Autodesk Inventor part; units mm, degrees
ref_plane "YZ Plane" through (0, 0, 0) normal (1, 0, 0) x (0, 1, 0)
ref_plane "XZ Plane" through (0, 0, 0) normal (0, 1, 0) x (-1, 0, 0)
ref_plane "XY Plane" through (0, 0, 0) normal (0, 0, 1) x (1, 0, 0)
sketch "Sketch1" plane through (0, 0, 0) normal (0, 0, 1) x (1, 0, 0)
  line L0 (0, 0) -> (50.8, 0)
  line L1 (50.8, 0) -> (50.8, 107.95)
  line L2 (50.8, 107.95) -> (0, 107.95)
  line L3 (0, 107.95) -> (0, 0)
  dimension "d0" = 50.8
  dimension "d1" = 107.95
extrude "Plate1" add sketch "Sketch1" along normal blind 3.048
sketch "Sketch2" plane through (47.752, 107.95, 0) normal (1, 0, 0) x (0, 1, 0)
  line L0 (-107.95, 0) -> (0, 0)
  line L1 (0, 0) -> (0, 76.2)
  line L2 (0, 76.2) -> (-107.95, 76.2)
  line L3 (-107.95, 76.2) -> (-107.95, 0)
edge flange "Flange1" height 76.2 angle 90 thickness 3.048 bend radius 3.048 thickness toward (1, 0, 0) relief tear relief width 3.048 relief depth 1.524 edges at (50.8, 53.975, 3.048) wall of the first edge with corners at (47.752, 0, 0) (47.752, 107.95, 0) (47.752, 107.95, 76.2) (47.752, 0, 76.2)
bend "Bend1"
corner "Corner1"
equation "\"d3\" = BendReliefWidth"
equation "\"d4\" = BendReliefDepth"
equation "\"d5\" = MinimumRemnant"
equation "\"d6\" = BendRadius"
equation "\"d9\" = BendRadius"
equation "\"d10\" = CornerReliefSize"
equation "\"d11\" = GapSize"
equation "\"d12\" = JacobiRadiusSize"
equation "\"BendRadius\" = Thickness"
equation "\"BendReliefWidth\" = Thickness"
equation "\"BendReliefDepth\" = 0.5 * Thickness"
equation "\"CornerReliefSize\" = 4 * Thickness"
equation "\"MinimumRemnant\" = 2 * Thickness"
equation "\"TransitionRadius\" = BendRadius"
equation "\"JacobiRadiusSize\" = BendRadius"
equation "\"GapSize\" = Thickness"
equation "\"d2\" = BendRadius"
properties part number "Claw - L bracket"
The listing builds one solid part. Answer for the finished solid, in the listing's coordinates (mm). A direction names the side the tool comes from. Coordinates: 2 decimals unless noted, no trailing zeros. Write each loop counter-clockwise with the first axis right and the second up, starting at its lowest first coordinate (ties: lowest second). Pieces come first, ordered by that corner, then holes. Notation, with made-up numbers: M 26.25,28.25 L 75.25,28.25 A17 cw 75.25,49.25 Z; hole C -13.5,50 d1. An arc over 180 degrees is marked long. Use one line per item in the form item = value.
Item 1: Find section B-B, the plane x = 15.5. Give the vertices of the cut face in (y, z).
Model answer:
outline = M 0,0 L 107.95,0 L 107.95,3.05 L 0,3.05 Z
Item 2: Find section A-A, the plane y = 101.5. Give the vertices of the cut face in (x, z), plus the area to 3 significant figures.
Model answer:
outline = M 0,0 L 44.7,0 A6.1 ccw 50.8,6.1 L 50.8,76.2 L 47.75,76.2 L 47.75,6.1 A3.05 cw 44.7,3.05 L 0,3.05 Z
area = 372 mm2
Item 3: Find section C-C, the plane z = 46.5. Give the vertices of the cut face in (x, y), plus the area to 3 significant figures.
Model answer:
outline = M 47.75,0 L 50.8,0 L 50.8,107.95 L 47.75,107.95 Z
area = 329 mm2
Item 4: Given P1, Ø10, axis at x = 42.5, y = 75, coming from the +Z side; P2, Ø8, axis at x = 5, y = 21, coming from the +Z side, each flat-ended and moving along its own axis, determine where each tip first touches the part or whether it passes through.
Model answer:
P1 = 4.88
P2 = 3.05
Item 5: For faces 1 (the face through (47.752, 55, 41)), 2 (the face through (50.8, 55, 42)), determine the directions among +Z, -Z, +X, -X, +Y, -Y from which every point of the face is accessible in a straight line to the end or side of a thin tool.
Model answer:
face_1 = +Z, -X, +Y, -Y
face_2 = +Z, -Z, +X, +Y, -Y
Item 6: Find the intervals of material crossed by probe 1 along X at (y, z) = (83, 56); probe 2 along Z at (x, y) = (45, 78); probe 3 along Z at (x, y) = (18, 66.5), in increasing order.
Model answer:
probe_1 = 47.75 to 50.8
probe_2 = 0.01 to 3.06
probe_3 = 0 to 3.05
